Can you work these out from the model? Positions are in its coordinate system, mm. A direction names the side the tool comes from. Coordinates: 2 decimals unless noted, no trailing zeros. Order: outer loops, then holes, each group sorted by start corner. A loop starts at its lowest first (then second) coordinate and runs counter-clockwise, first axis right, second up. Notation, with made-up numbers: (42, 6) - (52, 6) arc R15 ccw to (52, 29) - close; hole circle Ø11 at (86.25, -12.75). An arc over 180 degrees is marked (long way). Return JSON: item names as keys, results as strings. Group by question number.
1) For pin 1 Ø6 at (x, z) = (-21, 6.5) entering from -Y; pin 2 Ø2 at (y, z) = (-9.5, 11.5) entering from +X; pin 3 Ø1.9 at (x, z) = (20, 10) entering from -Y; pin 4 Ø5 at (x, z) = (12.5, 9) entering from -Y, each with a flat end and sliding along its axis, tell me the tip position at first contact or that it passes through.
2) If we mould it in two halves opening along X, with no side actions, what happens to faces 1 (the face through (24.1, -2.48, 19.14)), 2 (the face through (-20.35, -2.52, 8.44)), 3 (the face through (-18, -1, 10))? For each: pulls with the +X half, pulls with the -X half, needs draft (parallel to the pull), parting line crosses it, or undercut.
3) Imagine slicing it at A-A (y = -2.5). Write out the boundary of the cut face in (x, z).
4) If I drill on line 1 along Z through (x, y) = (20, -2.2); line 2 along Y through (x, z) = (18.5, 17.75); line 3 along Y through (x, z) = (0, 14.5), over which ranges is the centre line in solid material (lowest first)?
5) Imagine slicing it at C-C (z = 13.5). Write out the boundary of the cut face in (x, y).
6) Imagine slicing it at D-D (y = -10.5). Write out the boundary of the cut face in (x, z), and give its area (3 significant figures).
7) Imagine slicing it at B-B (x = -20). Write out the boundary of the cut face in (y, z), and give its area (3 significant figures).
8) Which directions (+Z, -Z, +X, -X, +Y, -Y) give clear straight access to the entire face, cutting with the end or side of a thin tool? Please do faces 4 (the face through (18, -4, 10)), 5 (the face through (-18, -4, 10)), 6 (the face through (-25, -2, 10)).
```python
from build123d import *

# Parameters (mm, degrees)
BOSS_EXTRUDE1_DEPTH = 20
SKETCH2_R           = 1.6
CUT_EXTRUDE1_DEPTH  = 20
FILLET1_R           = 3


with BuildPart() as part:
    # Sketch1 → Boss-Extrude1 (new body)
    with BuildSketch(Plane.XY):
        with BuildLine():
            Line((-10.95445115, -1), (-13.964240044, -1))
            ThreePointArc((-13.964240044, -1), (-13.772253627, -2.514961237), (-13.416407865, -4))
            ThreePointArc((-13.416407865, -4), (0, -14), (13.416407865, -4))
            ThreePointArc((13.416407865, -4), (13.772253627, -2.514961237), (13.964240044, -1))
            Line((13.964240044, -1), (10.95445115, -1))
            ThreePointArc((10.95445115, -1), (0, -11), (-10.95445115, -1))
        make_face()
        with BuildLine():
            Line((-13.964240044, -1), (-25, -1))
            Line((-25, -1), (-25, -4))
            Line((-25, -4), (-13.416407865, -4))
            ThreePointArc((-13.416407865, -4), (-13.772253627, -2.514961237), (-13.964240044, -1))
        make_face()
        with BuildLine():
            Line((25, -1), (13.964240044, -1))
            ThreePointArc((13.964240044, -1), (13.772253627, -2.514961237), (13.416407865, -4))
            Line((13.416407865, -4), (25, -4))
            Line((25, -4), (25, -1))
        make_face()
    extrude(amount=BOSS_EXTRUDE1_DEPTH)

    # Sketch2 → Cut-Extrude1 (cut)
    with BuildSketch(Plane.XZ.offset(4)):
        with Locations((-20, 10)):
            Circle(SKETCH2_R)
    cut_extrude1 = extrude(amount=-CUT_EXTRUDE1_DEPTH, mode=Mode.SUBTRACT)

    # Mirror1: Cut-Extrude1 across plane
    add(cut_extrude1.mirror(Plane(origin=(0, 0, 0), x_dir=(0, 0, 1), z_dir=(1, 0, 0))), mode=Mode.SUBTRACT)

    # Fillet1
    fillet1_edges = [part.edges().sort_by_distance(p)[0] for p in [
        (-25, -2.5, 0),
        (-25, -2.5, 20),
        (25, -2.5, 20),
        (25, -2.5, 0),
    ]]
    fillet(fillet1_edges, radius=FILLET1_R)


solid = part.part
```
Calculated:
{
 "1": {"pin 1": "y = -4", "pin 2": "x = 11.12", "pin 3": "through", "pin 4": "y = -9.8"},
 "2": {"face 1": "pulls with the +X half", "face 2": "undercut", "face 3": "needs draft"},
 "3": {"outline": "(-25, 3) arc R3 ccw to (-22, 0) - (-10.71, 0) - (-10.71, 20) - (-22, 20) arc R3 ccw to (-25, 17) - close; (10.71, 0) - (22, 0) arc R3 ccw to (25, 3) - (25, 17) arc R3 ccw to (22, 20) - (10.71, 20) - close; hole circle Ø3.2 at (-20, 10); hole circle Ø3.2 at (20, 10)"},
 "4": {"line 1": "0 to 8.4, 11.6 to 20", "line 2": "-4 to -1", "line 3": "-14 to -11"},
 "5": {"outline": "(-25, -4) - (-13.42, -4) arc R14 ccw to (13.42, -4) - (25, -4) - (25, -1) - (10.95, -1) arc R11 cw to (-10.95, -1) - (-25, -1) - close"},
 "6": {"outline": "(-9.26, 0) - (-3.28, 0) - (-3.28, 20) - (-9.26, 20) - close; (3.28, 0) - (9.26, 0) - (9.26, 20) - (3.28, 20) - close", "area": "239 mm2"},
 "7": {"outline": "(-4, 0) - (-1, 0) - (-1, 8.4) - (-4, 8.4) - close; (-4, 11.6) - (-1, 11.6) - (-1, 20) - (-4, 20) - close", "area": "50.4 mm2"},
 "8": {"face 4": "+Z, -Z, +X, -Y", "face 5": "+Z, -Z, -X, -Y", "face 6": "+Z, -Z, -X, +Y, -Y"}
}
